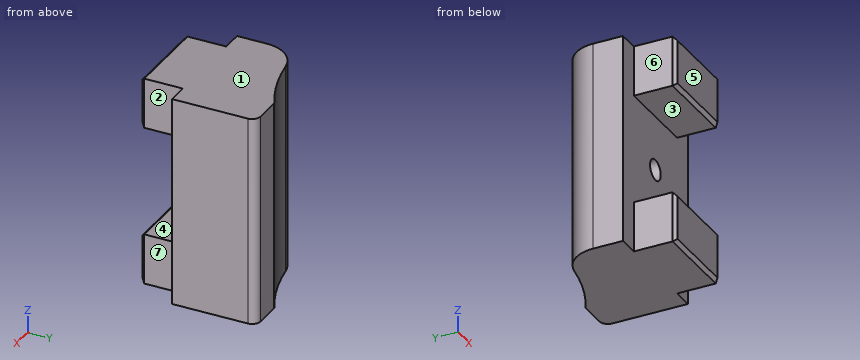
Autodesk Inventor part; units mm, degrees
ref_plane "YZ Plane" through (0, 0, 0) normal (1, 0, 0) x (0, 1, 0)
ref_plane "XZ Plane" through (0, 0, 0) normal (0, 1, 0) x (-1, 0, 0)
ref_plane "XY Plane" through (0, 0, 0) normal (0, 0, 1) x (1, 0, 0)
sketch "Skizze1" plane through (0, 0, 0) normal (0, 0, 1) x (1, 0, 0)
  circle A0 centre (0, 0) radius 22.75
  line L0 (0, -22.75) -> (0, -30)
  line L1 (0, -30) -> (15, -30)
  line L2 (15, -30) -> (15, -17.1045)
  line L3 (7.5, -17.7699) -> (7.5, -35.7566) construction
  line L4 (10.8426, -20) -> (15, -20)
  point P0 (7.5, -21.4782)
  dimension "d0" = 45.5
  dimension "d1" = 15
  dimension "d2" = 0
  dimension "d3" = 7.5
  dimension "d27" = 30
  dimension "d28" = 10
extrude "Extrusion1" add sketch "Skizze1" along normal blind 25 contours A0 L4 L2 L1 L0
fillet "Rundung1" radius 4 1 edges at (0, -22.75, 12.5)
sketch "Skizze2" plane through (0, -30, 0) normal (0, -1, 0) x (1, 0, 0)
  line L0 (2.5, 25) -> (12.5, 25)
  line L1 (12.5, 25) -> (12.5, 19)
  line L2 (12.5, 19) -> (2.5, 19)
  line L3 (2.5, 19) -> (2.5, 25)
  line L4 (2.5, 6) -> (12.5, 6)
  line L5 (12.5, 6) -> (12.5, 0)
  line L6 (12.5, 0) -> (2.5, 0)
  line L7 (2.5, 0) -> (2.5, 6)
  line L8 (7.5, 27.4511) -> (7.5, -5.4268) construction
  line L9 (0, 0) -> (0, 25)
  line L10 (0, 25) -> (15, 25)
  line L11 (0, 0) -> (15, 0)
  dimension "d8" = 6
  dimension "d9" = 6
  dimension "d10" = 10
  dimension "d11" = 7.5
extrude "Extrusion2" add sketch "Skizze2" along normal blind 5
sketch "Skizze3" plane through (0, -30, 0) normal (0, -1, 0) x (1, 0, 0)
  line L0 (0, 0) -> (0, 25)
  line L1 (2.5, 0) -> (12.5, 0)
  point P0 (7.5, 12.5)
  dimension "d25" = 7.5
  dimension "d26" = 12.5
hole "Bohrung1" at (7.5, -30, 12.5) direction (0, 1, 0) diameter 2.459 depth 6 tip angle 118
fillet "Rundung2" radius 1 1 edges at (15, -20, 12.5)
chamfer "Fase1" distance 0.4 angle 45 8 edges at (7.5, -35, 25) (2.5, -35, 22) (7.5, -35, 19) (12.5, -35, 22) (12.5, -35, 3) (7.5, -35, 6) (2.5, -35, 3) (7.5, -35, 0)
properties part number "103.020.01_Positionsausgleich" material "Polypropylen"
For this review, take the finished solid that the model builds, in its own axes (mm). Face numbers are marked on the shaded views. A direction names the side the tool comes from. Round coordinates to 2 decimals unless told otherwise and drop trailing zeros. Loops run counter-clockwise (first coordinate to the right, second up) from the corner with the lowest first, then second, coordinate; pieces in that order, holes last. Notation, with made-up numbers: (6, 29) - (53, 29) arc R12 ccw to (53, 52) - close; hole circle Ø5 at (46, 58). An arc over 180 degrees is marked (long way). Use one line per item in the form item = value.
1) Tool access review of the marked faces 5, 6 and 7: name each direction out of +Z, -Z, +X, -X, +Y, -Y from which nothing blocks a thin tool from reaching the whole face with its end or side.
Solutions:
face_5 = +Z, -Z, +X, -X, -Y
face_6 = +Z, -Z, -X, -Y
face_7 = +Z, -Z, +X, -Y
2) We need section A-A on z = 15.75. Write out the cut boundary in (x, y), then the cut area to 3 significant figures.
Solutions:
outline = (0, -30) - (15, -30) - (15, -21) arc R1 ccw to (14, -20) - (10.84, -20) arc R22.75 cw to (3.4, -22.49) arc R4 ccw to (0, -26.45) - close
area = 127 mm2
3) Clearance check with flat-ended pins moving along their axes: P1, Ø5, axis at y = -33, z = 1.5, coming from the -X side; P2, Ø1.4, axis at y = -31, z = 2, coming from the +X side; P3, Ø3, axis at x = 8.5, z = 9.5, coming from the -Y side. State where each tip first meets the part, or that it passes through.
Solutions:
P1 = 2.5
P2 = 12.5
P3 = -30
4) We need section C-C on x = 4.5. Write out the cut boundary in (y, z), then the cut area to 3 significant figures.
Solutions:
outline = (-35, 0.4) - (-34.6, 0) - (-22.3, 0) - (-22.3, 25) - (-34.6, 25) - (-35, 24.6) - (-35, 19.4) - (-34.6, 19) - (-30, 19) - (-30, 6) - (-34.6, 6) - (-35, 5.6) - close
area = 252 mm2
5) Mouldability with a two-part tool opening along Z and no side actions: class the marked faces 1, 2, 3 and 4 as pulls with the +Z half, pulls with the -Z half, needs draft (parallel to the pull), parting line crosses it, or undercut.
Solutions:
face_1 = pulls with the +Z half
face_2 = needs draft
face_3 = undercut
face_4 = undercut
6) Wall thickness on probe 1 along X at (y, z) = (-27, 12.5); probe 2 along Z at (x, y) = (11.75, -31); probe 3 along Z at (x, y) = (7, -25.75): over which ranges is each line inside the solid? List them lowest first.
Solutions:
probe_1 = 0 to 6.27, 8.73 to 15
probe_2 = 0 to 6, 19 to 25
probe_3 = 0 to 11.38, 13.62 to 25
7) We need section B-B on y = -25.5. Write out the cut boundary in (x, z), then the cut area to 3 significant figures.
Solutions:
outline = (0.11, 0) - (15, 0) - (15, 25) - (0.11, 25) - close; hole circle Ø2.46 at (7.5, 12.5)
area = 367 mm2
8) We need section D-D on z = 23.25. Write out the cut boundary in (x, y).
Solutions:
outline = (0, -30) - (2.5, -30) - (2.5, -34.6) - (2.9, -35) - (12.1, -35) - (12.5, -34.6) - (12.5, -30) - (15, -30) - (15, -21) arc R1 ccw to (14, -20) - (10.84, -20) arc R22.75 cw to (3.4, -22.49) arc R4 ccw to (0, -26.45) - close
